Geometry: see drawing. Coordinates: mm, zero at the bounding-box minimum. A direction names the side the tool comes from. Coordinates: 2 decimals unless noted, no trailing zeros. Write each loop counter-clockwise with the first axis right and the second up, starting at its lowest first coordinate (ties: lowest second). Pieces come first, ordered by that corner, then holes. Notation, with made-up numbers: M 20,84 L 24,84 A30 cw 24,118 Z; hole C 38,-14 d8. An arc over 180 degrees is marked long. Write item = value, one per line. Start each with the question number.
1. Pin query (flat end, axial travel): pin 1 Ø7.5 at (x, y) = (4.5, 8) entering from -Z; pin 2 Ø3 at (y, z) = (20.5, 2) entering from -X; pin 3 Ø2 at (x, y) = (3, 3) entering from -Z. Return the tip coordinate at first contact, or that it passes through.
2. Pull-direction query (Y, two-part tool) for the marked faces 3, 4 and 5; classes: pulls with the +Y half, pulls with the -Y half, needs draft (parallel to the pull), parting line crosses it, or undercut.
3. Section query B-B (z = 9.75). Output: boundary loops of the cut face in (x, y) (3 decimals), then the cut area to 3 significant figures.
4. Section query A-A (x = 7.5). Output: boundary loops of the cut face in (y, z) (1 decimal), then the cut area to 3 significant figures.
5. Line query: line 1 along Z through (x, y) = (10.75, 11); line 2 along Y through (x, z) = (5.5, 5.5); line 3 along X through (y, z) = (22.5, 2). Output: solid intervals per line, ascending.
6. Section query C-C (y = 7). Output: boundary loops of the cut face in (x, z), then the cut area to 3 significant figures.
7. Access query for the marked faces 1 and 2. Directions: +Z, -Z, +X, -X, +Y, -Y. A direction counts if a zero-diameter tool reaches every point of the face in a straight line with its end or side. Return the directions, or none.
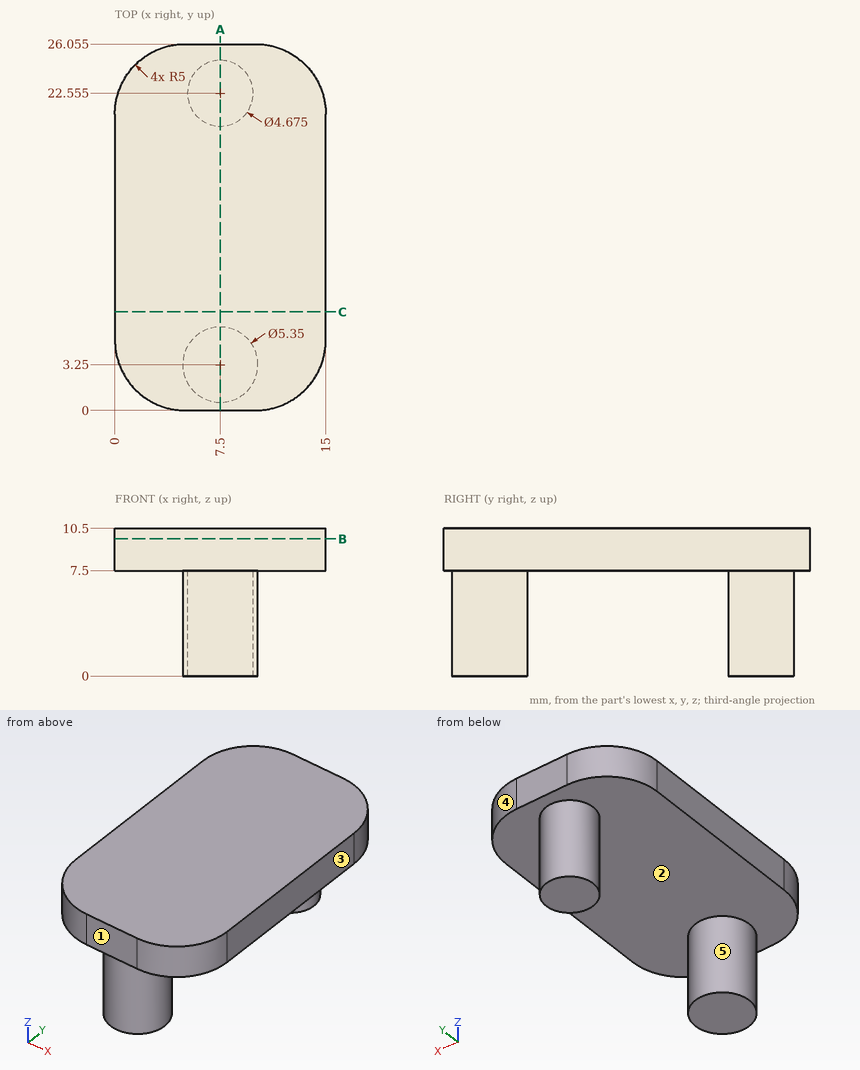
Results are:
q1.pin_1 = 0
q1.pin_2 = 5.23
q1.pin_3 = 7.5
q2.face_3 = needs draft
q2.face_4 = pulls with the +Y half
q2.face_5 = undercut
q3.outline = M 0,5 A5 ccw 5,0 L 10,0 A5 ccw 15,5 L 15,21.055 A5 ccw 10,26.055 L 5,26.055 A5 ccw 0,21.055 Z
q3.area = 369 mm^2
q4.outline = M 0,7.5 L 0.6,7.5 L 0.6,0 L 5.9,0 L 5.9,7.5 L 20.2,7.5 L 20.2,0 L 24.9,0 L 24.9,7.5 L 26.1,7.5 L 26.1,10.5 L 0,10.5 Z
q4.area = 153 mm^2
q5.line_1 = 7.5 to 10.5
q5.line_2 = 1.47 to 5.03, 21.35 to 23.76
q5.line_3 = 5.16 to 9.84
q6.outline = M 0,7.5 L 15,7.5 L 15,10.5 L 0,10.5 Z
q6.area = 45.0 mm^2
q7.face_1 = +Z, -Z, +X, -X, -Y
q7.face_2 = -Z
